The model under review builds one solid part; all positions refer to its coordinate system, in mm. A direction names the side the tool comes from. Round coordinates to 2 decimals unless told otherwise and drop trailing zeros. Order: outer loops, then holes, each group sorted by start corner. A loop starts at its lowest first (then second) coordinate and runs counter-clockwise, first axis right, second up. Notation, with made-up numbers: M 83,-9.75 L 132,-9.75 A20 ccw 132,28.25 Z; hole C 16.5,72 d2. An arc over 180 degrees is marked long. Answer as CSV lines item,"result". Start each with the question number.
from build123d import *

# Parameters (mm, degrees)
SKETCH_R         = 6
PAD_DEPTH        = 6.35
PAD001_DEPTH     = 14.351
HOLE_D           = 3.4
HOLE_CSINK_D     = 6.7
HOLE_CSINK_ANGLE = 90


with BuildPart() as part:
    # Sketch → Pad (new body)
    with BuildSketch(Plane.XZ):
        with BuildLine():
            ThreePointArc((21.388901, 18.814664), (-9.37148, 32.701744), (-10.552559, -1.027429))
            ThreePointArc((-4.298157, -14.707017), (-5.620109, -7.04185), (-10.552559, -1.027429))
            Line((-4.298157, -14.707017), (-4.826001, -20.740309))
            ThreePointArc((-4.826001, -20.740309), (-3.654583, -23.388806), (-0.789818, -23.812922))
            Line((-0.789818, -23.812922), (24.510486, -14.384528))
            ThreePointArc((24.510486, -14.384528), (26.0609, -13.073491), (26.421251, -11.075305))
            Line((26.421251, -11.075305), (21.388901, 18.814664))
        make_face()
        with Locations((8.324277, 14.830928)):
            Circle(SKETCH_R, mode=Mode.SUBTRACT)
    extrude(amount=PAD_DEPTH)

    # Sketch001 (on Face10 of Pad) → Pad001 (join)
    with BuildSketch(Plane.XZ.offset(6.35)):
        with BuildLine():
            ThreePointArc((-2.885017, -18.190632), (-4.648562, -22.049376), (-0.789818, -23.812922))
            Line((-0.789818, -23.812922), (24.510486, -14.384528))
            ThreePointArc((24.510486, -14.384528), (26.274032, -10.525783), (22.415287, -8.762238))
            Line((-2.885017, -18.190632), (22.415287, -8.762238))
        make_face()
    extrude(amount=PAD001_DEPTH)

    # Hole (through all)
    with Locations(Plane(origin=(0, 0, 0), x_dir=(1, 0, 0), z_dir=(0, 1, 0))):
        with Locations((-1.837417, 21.001777), (23.462887, 11.573383), (15.398685, -21.991601), (2.701828, -30.882036), (-11.345943, -24.331453), (-12.696857, -8.890435), (0, 0), (14.047771, -6.550583)):
            CounterSinkHole(HOLE_D / 2, HOLE_CSINK_D / 2, counter_sink_angle=HOLE_CSINK_ANGLE)


solid = part.part
Item 1: Consider section D-D (y = -13). State the section outline as (x, z) points.
Item 2: Tool access review of faces 4 (the flat face through (-4.56, -3.13, -17.68)), 5 (the flat face through (3, 0, 7)): name each direction out of +Z, -Z, +X, -X, +Y, -Y from which nothing blocks a thin tool from reaching the whole face with its end or side.
Item 3: For pin 1 (14 mm diameter, centred on x = 8.32, z = 14.83, fed in from -Y); pin 2 (5.5 mm diameter, centred on x = 0, z = 0, fed in from +Y); pin 3 (4 mm diameter, centred on x = 2.7, z = 30.88, fed in from +Y), all flat-tipped, find the tip position at first contact; note any pin that passes through.
Item 4: Wall thickness on probe 1 along Y at (x, z) = (20, 2); probe 2 along Z at (x, y) = (-10.5, -4); probe 3 along X at (y, z) = (-3.25, 31): over which ranges is each line inside the solid? List them lowest first. Write a range as [from, to].
Item 5: The part is to be moulded in two halves that separate along Z. For faces 1 (the flat face through (23.94, -3.13, 3.66)), 2 (the cylindrical face through (0.37, -4.03, 1.66)), 3 (the flat face through (11, -20.701, -16)), say which applies: +Z half, -Z half, draft (parallel to the pull), parting line (faces both ways), or undercut.
Item 6: Consider section A-A (x = 10). State the section outline as (y, z) points.
Item 7: Consider section C-C (y = -3). State how many separate pieces and enclosed holes the cut face has, and give its area (3 significant figures).
Item 8: Consider section B-B (z = 0). State the section outline as (x, y) points.
Reported:
1,outline,"M -2.89,-18.19 A3 ccw -0.79,-23.81 L 24.51,-14.38 A3 ccw 22.42,-8.76 Z; hole C -1.84,-21 d3.4; hole C 23.46,-11.57 d3.4"
2,face 4,"-X, +Y, -Y"
2,face 5,"+Z, -Z, +X, -X, +Y"
3,pin 1,"stops at y = -6.35"
3,pin 2,"stops at y = -0.6"
3,pin 3,"stops at y = -1.35"
4,probe 1,"y = [-6.35, 0]"
4,probe 2,"z = [-1.07, 22.86], [25.81, 31.95]"
4,probe 3,"x = [-11.72, 1.01], [4.4, 14.42]"
5,face 1,"+Z half"
5,face 2,"undercut"
5,face 3,"draft"
6,outline,"M -20.7,-19.79 L 0,-19.79 L 0,9.07 L -6.35,9.07 L -6.35,-13.39 L -20.7,-13.39 Z; M -6.35,20.59 L 0,20.59 L 0,33.83 L -6.35,33.83 Z"
7,separate pieces,"1"
7,enclosed holes,"9"
7,area,"1,700 mm²"
8,outline,"M -11.86,-6.35 L -1.7,-6.35 L -1.7,-1.65 L -3.35,0 L -11.86,0 Z; M 1.7,-6.35 L 24.56,-6.35 L 24.56,0 L 3.35,0 L 1.7,-1.65 Z"
